```python
from build123d import *

# Parameters (mm, degrees)
SKETCH1_W           = 10
SKETCH1_H           = 5
BOSS_EXTRUDE1_DEPTH = 3


with BuildPart() as part:
    # Sketch1 → Boss-Extrude1 (new body)
    with BuildSketch(Plane.XY):
        Polygon((90, 201.25), (0, 0), (85, 0), (85, 7.26), (95, 7.26), (95, 0), (180, 0), align=None)
        with Locations((90, 89.737444444)):
            Rectangle(SKETCH1_W, SKETCH1_H, mode=Mode.SUBTRACT)
    extrude(amount=BOSS_EXTRUDE1_DEPTH)


solid = part.part
```
Here's how the part is built. I have some questions about the finished solid (model axes, mm). Round coordinates to 2 decimals unless told otherwise and drop trailing zeros. Loops run counter-clockwise (first coordinate to the right, second up) from the corner with the lowest first, then second, coordinate; pieces in that order, holes last. Notation, with made-up numbers: (45.5, 42.5) -> (99.5, 42.5) arc R31 ccw to (99.5, 77.5) -> close; hole circle Ø9 at (65.25, -34). An arc over 180 degrees is marked (long way). Answer as CSV lines item,"result".
1. If I drill on L1, parallel to X at y = 144.5, z = 2.6; L2, parallel to X at y = 180, z = 1.45; L3, parallel to X at y = 90, z = 0.2, over which ranges is the centre line in solid material (lowest first)?
Final values:
L1,"x = 64.62 to 115.38"
L2,"x = 80.5 to 99.5"
L3,"x = 40.25 to 85, 95 to 139.75"
2. If we section it at C-C on x = 162: Please give me the cut outline in (y, z).
Final values:
outline,"(0, 0) -> (40.25, 0) -> (40.25, 3) -> (0, 3) -> close"
3. If we section it at B-B on y = 159: Please give me the cut outline in (x, z), plus the area to 3 significant figures.
Final values:
outline,"(71.11, 0) -> (108.89, 0) -> (108.89, 3) -> (71.11, 3) -> close"
area,"113 mm^2"
4. If we section it at A-A on z = 0.7: Please give me the cut outline in (x, y).
Final values:
outline,"(0, 0) -> (85, 0) -> (85, 7.26) -> (95, 7.26) -> (95, 0) -> (180, 0) -> (90, 201.25) -> close; hole (85, 87.24) -> (95, 87.24) -> (95, 92.24) -> (85, 92.24) -> close"
5. For pin 1 (1.5 mm diameter, centred on y = 5, z = 2, fed in from -X); pin 2 (1.5 mm diameter, centred on x = 91.5, z = 1, fed in from -Y); pin 3 (1.5 mm diameter, centred on y = 4.5, z = 1, fed in from +X); pin 4 (1.5 mm diameter, centred on x = 66.5, z = 1, fed in from -Y), each with a flat end and sliding along its axis, tell me the tip position at first contact or that it passes through.
Final values:
pin 1,"stops at x = 1.9"
pin 2,"stops at y = 7.26"
pin 3,"stops at x = 178.32"
pin 4,"stops at y = 0"
